```python
from build123d import *

# Parameters (mm, degrees)
SKETCH1_W               = 40
SKETCH1_H               = 34.7
BOSS_EXTRUDE1_DEPTH     = 20
SKETCH2_R               = 8.1
CUT_EXTRUDE1_DEPTH      = 12.7
SKETCH5_W               = 11.15
SKETCH5_H               = 40
CUT_EXTRUDE5_DEPTH      = 22
SKETCH9_R               = 8.1
SKETCH9_R_2             = 6.1
BOSS_EXTRUDE2_DEPTH     = 5.7
CUT_EXTRUDE6_DEPTH      = 57.604681952
CUT_EXTRUDE6_DEPTH_BACK = 57.604681952
SKETCH10_W              = 12
SKETCH10_H              = 40
SKETCH11_R              = 1.95
CUT_EXTRUDE7_DEPTH      = 8
CHAMFER1_SIZE           = 1
SKETCH12_R              = 1.95
CUT_EXTRUDE8_DEPTH      = 54.889609545
CHAMFER2_SIZE           = 1
SKETCH15_R              = 1.95
CUT_EXTRUDE11_DEPTH     = 10
CHAMFER3_SIZE           = 1
CHAMFER7_SIZE           = 3


with BuildPart() as part:
    # Sketch1 → Boss-Extrude1 (new body)
    with BuildSketch(Plane(origin=(0, 0, 0), x_dir=(0, 0, -1), z_dir=(1, 0, 0))):
        with Locations((20, 17.35)):
            Rectangle(SKETCH1_W, SKETCH1_H)
    extrude(amount=-BOSS_EXTRUDE1_DEPTH)

    # Sketch2 → Cut-Extrude1 (cut)
    with BuildSketch(Plane(origin=(0, 34.7, 0), x_dir=(1, 0, 0), z_dir=(0, 1, 0))):
        with Locations((0.3, 20)):
            Circle(SKETCH2_R)
    extrude(amount=-CUT_EXTRUDE1_DEPTH, mode=Mode.SUBTRACT)

    # Sketch5 → Cut-Extrude5 (cut)
    with BuildSketch(Plane.XZ):
        with Locations((-5.575, -20)):
            Rectangle(SKETCH5_W, SKETCH5_H)
    extrude(amount=-CUT_EXTRUDE5_DEPTH, mode=Mode.SUBTRACT)

    # Cut-Loft1: read off the stored shape, not the designer's step
    # Cut-Loft1: loft between two sections, ruled curve by curve
    cut_loft1_from = [
        Edge.make_bspline([(11.243514961, 28.316114759, -40), (10.488221253, 28.870573657, -40), (9.673151561, 29.382537078, -40), (7.939112522, 30.28953078, -40), (7.020163395, 30.684407436, -40), (5.104947281, 31.329224581, -40), (4.108776624, 31.579024462, -40), (2.074994957, 31.914454558, -40), (1.037543565, 32, -40), (-1.037543565, 32, -40), (-2.074994957, 31.914454558, -40), (-4.108776624, 31.579024462, -40), (-5.104947281, 31.329224581, -40), (-7.020163395, 30.684407436, -40), (-7.939112522, 30.28953078, -40), (-9.673151561, 29.382537078, -40), (-10.488221253, 28.870573657, -40), (-11.243514961, 28.316114759, -40)], [0, 0, 0, 0, 0.125, 0.125, 0.25, 0.25, 0.375, 0.375, 0.5, 0.5, 0.625, 0.625, 0.75, 0.75, 0.875, 0.875, 1, 1, 1, 1], 3),
        Edge.make_bspline([(-11.243514961, 28.316114759, -40), (-12.272389396, 27.560821051, -40), (-13.278735727, 26.661602289, -40), (-15.139556406, 24.56538073, -40), (-15.993134823, 23.367779698, -40), (-17.42758787, 20.71689046, -40), (-18.007136515, 19.263731202, -40), (-18.79386095, 16.206568982, -40), (-19, 14.603683637, -40), (-19, 11.396316363, -40), (-18.79386095, 9.793431018, -40), (-18.007136515, 6.736268798, -40), (-17.42758787, 5.28310954, -40), (-15.993134823, 2.632220302, -40), (-15.139556406, 1.43461927, -40), (-13.278735727, -0.661602289, -40), (-12.272389396, -1.560821051, -40), (-11.243514961, -2.316114759, -40)], [0, 0, 0, 0, 0.125, 0.125, 0.25, 0.25, 0.375, 0.375, 0.5, 0.5, 0.625, 0.625, 0.75, 0.75, 0.875, 0.875, 1, 1, 1, 1], 3),
        Edge.make_line((-11.243514961, -2.316114759, -40), (11.243514961, 28.316114759, -40)),
    ]
    cut_loft1_to = [
        Edge.make_bspline([(11.85, 22, -28), (10.891666667, 22, -28), (9.933333333, 22, -28), (8.016666667, 22, -28), (7.058333333, 22, -28), (5.141666667, 22, -28), (4.183333333, 22, -28), (2.266666667, 22, -28), (1.308333333, 22, -28), (-0.608333333, 22, -28), (-1.566666667, 22, -28), (-3.483333333, 22, -28), (-4.441666667, 22, -28), (-6.358333333, 22, -28), (-7.316666667, 22, -28), (-9.233333333, 22, -28), (-10.191666667, 22, -28), (-11.15, 22, -28)], [0, 0, 0, 0, 0.125, 0.125, 0.25, 0.25, 0.375, 0.375, 0.5, 0.5, 0.625, 0.625, 0.75, 0.75, 0.875, 0.875, 1, 1, 1, 1], 3),
        Edge.make_bspline([(-11.15, 22, -28), (-11.15, 20.694541399, -28), (-11.15, 19.389082798, -28), (-11.15, 16.778165596, -28), (-11.15, 15.472706995, -28), (-11.15, 12.861789793, -28), (-11.15, 11.556331192, -28), (-11.15, 8.94541399, -28), (-11.15, 7.639955389, -28), (-11.15, 5.029038187, -28), (-11.15, 3.723579586, -28), (-11.15, 1.112662384, -28), (-11.15, -0.192796217, -28), (-11.15, -2.803713419, -28), (-11.15, -4.10917202, -28), (-11.15, -6.720089222, -28), (-11.15, -8.025547823, -28), (-11.15, -9.331006424, -28)], [0, 0, 0, 0, 0.125, 0.125, 0.25, 0.25, 0.375, 0.375, 0.5, 0.5, 0.625, 0.625, 0.75, 0.75, 0.875, 0.875, 1, 1, 1, 1], 3),
        Edge.make_line((-11.15, -9.331006424, -28), (11.85, 22, -28)),
    ]
    cut_loft1 = Solid(Shell([*[Face.make_surface_from_curves(cut_loft1_from[k], cut_loft1_to[k]) for k in range(3)], Face(Wire(cut_loft1_from)), Face(Wire(cut_loft1_to))]))
    add(cut_loft1, mode=Mode.SUBTRACT)

    # Sketch9 → Boss-Extrude2 (add)
    with BuildSketch(Plane(origin=(0, 31, 0), x_dir=(1, 0, 0), z_dir=(0, 1, 0))):
        with Locations((0.3, 20)):
            Circle(SKETCH9_R)
        with Locations(Location((0.3, 20, 0), (0, 0, 270))):
            Circle(SKETCH9_R_2, mode=Mode.SUBTRACT)
    extrude(amount=-BOSS_EXTRUDE2_DEPTH)

    # Sketch10 → Cut-Extrude6 (cut, two sides: drawn at the far end of the back side and taken through both)
    with BuildSketch(Plane(origin=(0, 0, 0), x_dir=(1, 0, 0), z_dir=(0, 1, 0)).offset(-CUT_EXTRUDE6_DEPTH_BACK)):
        with Locations((6, 20)):
            Rectangle(SKETCH10_W, SKETCH10_H)
    extrude(amount=CUT_EXTRUDE6_DEPTH + CUT_EXTRUDE6_DEPTH_BACK, mode=Mode.SUBTRACT)

    # Sketch11 → Cut-Extrude7 (cut)
    with BuildSketch(Plane.XZ):
        with Locations(Location((-15.575, -13.907381515, 0), (0, 0, 270))):
            Circle(SKETCH11_R)
        with Locations(Location((-15.575, -26.092618485, 0), (0, 0, 270))):
            Circle(SKETCH11_R)
    extrude(amount=-CUT_EXTRUDE7_DEPTH, mode=Mode.SUBTRACT)

    # Chamfer1
    chamfer1_edges = [part.edges().sort_by_distance(p)[0] for p in [
        (-15.575, 0, -11.957381515),
        (-15.575, 0, -24.142618485),
    ]]
    chamfer(chamfer1_edges, length=CHAMFER1_SIZE)

    # Sketch12 → Cut-Extrude8 (cut, through all)
    with BuildSketch(Plane(origin=(-10, 0, 0), x_dir=(0, 0, -1), z_dir=(1, 0, 0))):
        with Locations(Location((9.907381515, 28.15, 0), (0, 0, 180))):
            Circle(SKETCH12_R)
        with Locations(Location((30.092618485, 28.15, 0), (0, 0, 180))):
            Circle(SKETCH12_R)
    extrude(amount=CUT_EXTRUDE8_DEPTH, mode=Mode.SUBTRACT)

    # Chamfer2
    chamfer2_edges = [part.edges().sort_by_distance(p)[0] for p in [
        (0, 28.15, -11.857381515),
        (0, 28.15, -32.042618485),
    ]]
    chamfer(chamfer2_edges, length=CHAMFER2_SIZE)

    # Sketch15 → Cut-Extrude11 (cut)
    with BuildSketch(Plane(origin=(0, 0, -40), x_dir=(-1, 0, 0), z_dir=(0, 0, -1))):
        with Locations((16, 29)):
            Circle(SKETCH15_R)
    extrude(amount=-CUT_EXTRUDE11_DEPTH, mode=Mode.SUBTRACT)

    # Chamfer3
    chamfer3_edges = [part.edges().sort_by_distance(p)[0] for p in [
        (-14.05, 29, -40),
    ]]
    chamfer(chamfer3_edges, length=CHAMFER3_SIZE)

    # Chamfer7
    chamfer7_edges = [part.edges().sort_by_distance(p)[0] for p in [
        (-20, 34.7, -20),
    ]]
    chamfer(chamfer7_edges, length=CHAMFER7_SIZE)


solid = part.part
```
Can you work these out from the model? Positions are in its coordinate system, mm. A direction names the side the tool comes from. Coordinates: 2 decimals unless noted, no trailing zeros. Order: outer loops, then holes, each group sorted by start corner. A loop starts at its lowest first (then second) coordinate and runs counter-clockwise, first axis right, second up.
1. For faces 4 (the face through (-11.15, 11, -14)), 5 (the face through (-16, 29, -30)), 6 (the face through (-5.56, 29.88, -9.01)), which set-ups out of +Z, -Z, +X, -X, +Y, -Y let a thin tool reach every point of the face, with its end or its side?
2. I'm going to push flat-ended pins straight in: pin 1 (6 mm diameter, centred on x = -5, z = -19.5, fed in from -Y); pin 2 (3.5 mm diameter, centred on x = -16, y = 29, fed in from -Z); pin 3 (2.5 mm diameter, centred on y = 28.15, z = -30.09, fed in from +X). Where does each tip first touch, or does it pass through?
3. I need wall thicknesses on line 1 (Y direction, x = -16, z = -32.75); line 2 (Z direction, x = -6.5, y = 28.15); line 3 (Y direction, x = -2, z = -2). Which ranges of each line are inside material? Lowest first, please.
4. Thinking about a two-plate mould opening in Y: for faces 1 (the face through (-16, 8, -26)), 2 (the face through (-10, 28, -10)), 3 (the face through (-12, 21, 0)), which applies, +Y half, -Y half, draft (parallel to the pull), parting line (faces both ways), or undercut?
5. If we section it at A-A (z = -20): Please give me the cut outline in (x, y).
6. If we section it at B-B (x = -9.5): Give the number of separate pieces and of enclosed holes in the cut face, then the cut area to 3 significant figures.
7. If we section it at C-C (z = -2.5): Please give me the cut outline in (x, y).
Entries:
1. face 4: +Z, -Z, +X, -Y
1. face 5: -Z
1. face 6: +X
2. pin 1: stops at y = 22
2. pin 2: stops at z = -30
2. pin 3: stops at x = -10
3. line 1: y = 0 to 27.05, 30.95 to 34.7
3. line 2: z = -36.4 to -32.04, -28.14 to -11.86, -7.96 to 0
3. line 3: y = 22 to 34.7
4. face 1: -Y half
4. face 2: undercut
4. face 3: draft
5. outline: (-20, 0) - (-11.15, 0) - (-11.15, 22) - (-7.8, 22) - (-7.8, 25.3) - (-5.8, 25.3) - (-5.8, 31) - (-7.8, 31) - (-7.8, 34.7) - (-17, 34.7) - (-20, 31.7) - close
6. separate pieces: 1
6. enclosed holes: 2
6. area: 440 mm2
7. outline: (-20, 0) - (-11.15, 0) - (-11.15, 22) - (0, 22) - (0, 34.7) - (-17, 34.7) - (-20, 31.7) - close
